from build123d import *

# Parameters (mm, degrees)
SKETCH1_W                                       = 63.5
SKETCH1_H                                       = 6.35
BOSS_EXTRUDE1_DEPTH                             = 50.8
BOSS_EXTRUDE2_DEPTH                             = 50.8
SKETCH10_W                                      = 6.604
SKETCH10_H                                      = 25.629031657
CUT_EXTRUDE1_DEPTH                              = 88.854357354
LPATTERN3_COUNT                                 = 2
LPATTERN3_PITCH                                 = 31.496
SKETCH11_R                                      = 4.09575
CUT_EXTRUDE2_DEPTH                              = 88.854357354
CBORE_FOR_10_SOCKET_HEAD_CAP_SCREW1_D           = 5.1054
CBORE_FOR_10_SOCKET_HEAD_CAP_SCREW1_CBORE_D     = 9.525
CBORE_FOR_10_SOCKET_HEAD_CAP_SCREW1_CBORE_DEPTH = 4.826
CBORE_FOR_10_SOCKET_HEAD_CAP_SCREW3_D           = 5.1054
CBORE_FOR_10_SOCKET_HEAD_CAP_SCREW3_CBORE_D     = 9.525
CBORE_FOR_10_SOCKET_HEAD_CAP_SCREW3_CBORE_DEPTH = 11.176


with BuildPart() as part:
    # Sketch1 → Boss-Extrude1 (new body)
    with BuildSketch(Plane(origin=(0, 0, 0), x_dir=(0, 0, -1), z_dir=(1, 0, 0))):
        with Locations((31.75, 3.175)):
            Rectangle(SKETCH1_W, SKETCH1_H)
    extrude(amount=-BOSS_EXTRUDE1_DEPTH)

    # Sketch2 → Boss-Extrude2 (add)
    with BuildSketch(Plane(origin=(0, 0, 0), x_dir=(0, 0, -1), z_dir=(1, 0, 0))):
        Polygon((0, 6.35), (0, 19.05), (12.7, 33.249031657), (50.8, 33.249031657), (63.5, 19.05), (63.5, 6.35), align=None)
    extrude(amount=-BOSS_EXTRUDE2_DEPTH)

    # Sketch10 → Cut-Extrude1 (cut, through all)
    with BuildSketch(Plane(origin=(0, 0, -63.5), x_dir=(-1, 0, 0), z_dir=(0, 0, -1))):
        with Locations((9.652, 20.434515829)):
            Rectangle(SKETCH10_W, SKETCH10_H)
    cut_extrude1 = extrude(amount=-CUT_EXTRUDE1_DEPTH, mode=Mode.SUBTRACT)

    # LPattern3: Cut-Extrude1 ×2
    with Locations(*[(-i * LPATTERN3_PITCH, 0, 0) for i in range(1, LPATTERN3_COUNT)]):
        add(cut_extrude1, mode=Mode.SUBTRACT)

    # Sketch11 → Cut-Extrude2 (cut, through all)
    with BuildSketch(Plane(origin=(0, 0, 0), x_dir=(0, 0, -1), z_dir=(1, 0, 0))):
        with Locations((22.86, 19.05)):
            Circle(SKETCH11_R)
        with Locations((40.64, 19.05)):
            Circle(SKETCH11_R)
    extrude(amount=-CUT_EXTRUDE2_DEPTH, mode=Mode.SUBTRACT)

    # CBORE for #10 Socket Head Cap Screw1 (through all)
    with Locations(Plane(origin=(0, 33.249031657, 0), x_dir=(1, 0, 0), z_dir=(0, 1, 0))):
        with Locations((-25.4, 31.75)):
            CounterBoreHole(CBORE_FOR_10_SOCKET_HEAD_CAP_SCREW1_D / 2, CBORE_FOR_10_SOCKET_HEAD_CAP_SCREW1_CBORE_D / 2, CBORE_FOR_10_SOCKET_HEAD_CAP_SCREW1_CBORE_DEPTH)

    # CBORE for #10 Socket Head Cap Screw3 (through all)
    with Locations(Plane(origin=(0, 33.02, 0), x_dir=(-1, 0, 0), z_dir=(0, 1, 0))):
        with Locations((25.4, -6.35), (25.4, -57.15)):
            CounterBoreHole(CBORE_FOR_10_SOCKET_HEAD_CAP_SCREW3_D / 2, CBORE_FOR_10_SOCKET_HEAD_CAP_SCREW3_CBORE_D / 2, CBORE_FOR_10_SOCKET_HEAD_CAP_SCREW3_CBORE_DEPTH)


solid = part.part
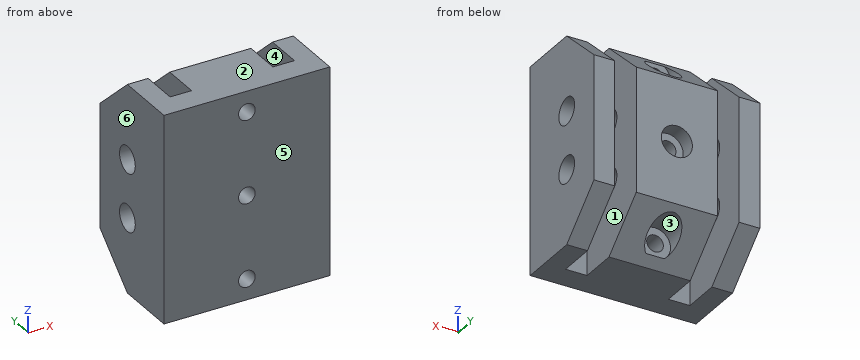
Input: part model. Units: mm. Frame: model coordinates. Face numbers are marked on the shaded views. A direction names the side the tool comes from. Give positions to 0.01 mm unless a question says otherwise; leave off trailing zeros. Write each loop counter-clockwise with the first axis right and the second up, starting at its lowest first coordinate (ties: lowest second). Pieces come first, ordered by that corner, then holes. Notation, with made-up numbers: M 59.5,46.25 L 114.5,46.25 A17 ccw 114.5,79.25 Z; hole C 69,60 d4. An arc over 180 degrees is marked long. Write item = value, one per line. Start each with the question number.
1) Cut plane C-C on z = -31.75. Return the cut outline in (x, y), then the cut area to 3 significant figures.
2) First-contact query: pin 1 Ø4 at (x, z) = (-8.5, -15.5) entering from +Y; pin 2 Ø4.5 at (x, z) = (-26, -6) entering from +Y; pin 3 Ø6 at (x, y) = (-39.5, 26.5) entering from +Z. Flat tips, straight axial feed; report the tip coordinate or a pass-through.
3) Cut plane B-B on z = -40.64. Return the cut outline in (x, y), then the cut area to 3 significant figures.
4) Material intervals for line 1 along Z through (x, y) = (-25.4, 13); line 2 along X through (y, z) = (20, -46); line 3 along Z through (x, y) = (-20.5, 19), sorted ascending. Write a range as [from, to].
5) Reachability of the marked faces 1, 2 and 3 from +Z, -Z, +X, -X, +Y, -Y: full face, straight path, thin tool, end or side. Return the list, or none.
6) Cut plane D-D on x = -36. Return the cut outline in (y, z), then the cut area to 3 significant figures.
7) Cut plane A-A on x = -25.4. Count the separate pieces of the cut face and the enclosed holes in it, then the cut area to 3 significant figures.
8) Draft query along X for the marked faces 4, 5 and 6. Return one class per face: +X half, -X half, draft (parallel to the pull), parting line (faces both ways), or undercut.
Solved:
q1.outline = M -50.8,0 L -27.95,0 L -27.95,28.42 L -30.16,28.42 L -30.16,33.25 L -37.85,33.25 L -37.85,7.62 L -44.45,7.62 L -44.45,33.25 L -50.8,33.25 Z; M -22.85,0 L 0,0 L 0,33.25 L -6.35,33.25 L -6.35,7.62 L -12.95,7.62 L -12.95,33.25 L -20.64,33.25 L -20.64,28.42 L -22.85,28.42 Z
q1.area = 1,160 mm2
q2.pin_1 = 7.62
q2.pin_2 = 21.84
q2.pin_3 = -4.42
q3.outline = M -50.8,0 L 0,0 L 0,14.95 L -6.35,14.95 L -6.35,7.62 L -12.95,7.62 L -12.95,14.95 L -37.85,14.95 L -37.85,7.62 L -44.45,7.62 L -44.45,14.95 L -50.8,14.95 Z; M -50.8,23.15 L -44.45,23.15 L -44.45,33.25 L -50.8,33.25 Z; M -37.85,23.15 L -12.95,23.15 L -12.95,33.25 L -37.85,33.25 Z; M -6.35,23.15 L 0,23.15 L 0,33.25 L -6.35,33.25 Z
q3.area = 1,040 mm2
q4.line_1 = [-63.5, -59.7], [-54.6, -34.3], [-29.2, -8.9], [-3.8, 0]
q4.line_2 = [-50.8, -44.45], [-37.85, -12.95], [-6.35, 0]
q4.line_3 = [-63.5, -44.74], [-36.54, -26.96], [-18.76, 0]
q5.face_1 = +Z, -Z, +Y
q5.face_2 = +Z, +X, -X, +Y, -Y
q5.face_3 = +Y
q6.outline = M 0,-63.5 L 19.05,-63.5 L 33.25,-50.8 L 33.25,-12.7 L 19.05,0 L 0,0 Z; hole C 19.05,-40.64 d8.19; hole C 19.05,-22.86 d8.19
q6.area = 1,830 mm2
q7.separate_pieces = 4
q7.enclosed_holes = 2
q7.area = 1,330 mm2
q8.face_4 = undercut
q8.face_5 = draft
q8.face_6 = -X half
